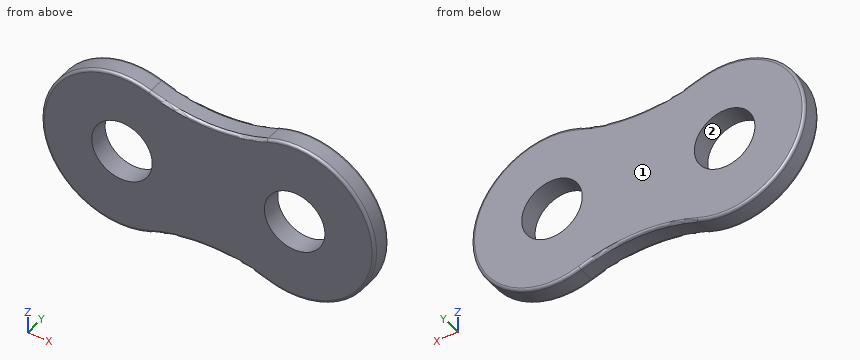
```python
from build123d import *

# Parameters (mm, degrees)
SZKIC1_R                    = 2.225
DODANIE_WYCI_GNI_CIE1_DEPTH = 1.5
ZAOKR_GLENIE1_R             = 0.2


with BuildPart() as part:
    # Szkic1 → Dodanie-wyciągnięcie1 (new body)
    with BuildSketch(Plane(origin=(0, 0, 0), x_dir=(1, 0, 0), z_dir=(0, 1, 0))):
        with BuildLine():
            ThreePointArc((2.036141304, 5.537520076), (-5.9, 0), (2.036141304, -5.537520076))
            ThreePointArc((2.036141304, -5.537520076), (6.35, -4.769554134), (10.663858696, -5.537520076))
            ThreePointArc((10.663858696, -5.537520076), (18.6, 0), (10.663858696, 5.537520076))
            ThreePointArc((10.663858696, 5.537520076), (6.35, 4.769554134), (2.036141304, 5.537520076))
        make_face()
        with Locations(Location((0, 0, 0), (0, 0, 270))):
            Circle(SZKIC1_R, mode=Mode.SUBTRACT)
        with Locations(Location((12.7, 0, 0), (0, 0, 270))):
            Circle(SZKIC1_R, mode=Mode.SUBTRACT)
    extrude(amount=DODANIE_WYCI_GNI_CIE1_DEPTH)

    # Zaokrąglenie1
    zaokr_glenie1_edges = [part.edges().sort_by_distance(p)[0] for p in [
        (6.35, 1.5, 4.769554134),
        (18.6, 1.5, 0),
        (6.35, 1.5, -4.769554134),
        (18.6, 0, 0),
        (6.35, 0, 4.769554134),
        (-5.9, 0, 0),
        (6.35, 0, -4.769554134),
        (-5.9, 1.5, 0),
    ]]
    fillet(zaokr_glenie1_edges, radius=ZAOKR_GLENIE1_R)


solid = part.part
```
Can you work these out from the model? Positions are in its coordinate system, mm. Face numbers are marked on the shaded views. Round coordinates to 2 decimals unless told otherwise and drop trailing zeros. Loops run counter-clockwise (first coordinate to the right, second up) from the corner with the lowest first, then second, coordinate; pieces in that order, holes last.
Item 1: Please list where these lines run through material, in increasing order: L1, parallel to X at y = 0.85, z = 0 (3 decimals); L2, parallel to Z at x = 13.5, y = 1.2; L3, parallel to Z at x = 13.75, y = 0.5.
Item 2: If we mould it in two halves opening along X, with no side actions, what happens to the marked faces 1 and 2? For each: +X half, -X half, draft (parallel to the pull), parting line (faces both ways), or undercut.
Item 3: Suppose I cut it at A-A, the plane y = 1. Write out the boundary of the cut face in (x, z) (3 decimals).
Item 4: Will these pins go through, and if not, where does the flat tip stop? pin 1 Ø6 at (x, z) = (4, -1.5) entering from -Y; pin 2 Ø2.5 at (x, z) = (0, 0) entering from +Y.
Item 5: Suppose I cut it at C-C, the plane z = -1.5. State how many separate pieces and enclosed holes the cut face has, then the cut area to 3 significant figures.
Item 6: Suppose I cut it at B-B, the plane z = 0. Write out the boundary of the cut face in (x, y) (3 decimals).
Reported:
1. L1: x = -5.9 to -2.225, 2.225 to 10.475, 14.925 to 18.6
1. L2: z = -5.85 to -2.08, 2.08 to 5.85
1. L3: z = -5.81 to -1.96, 1.96 to 5.81
2. face 1: draft
2. face 2: undercut
3. outline: (2.036, -5.538) arc R12.5 cw to (10.664, -5.538) arc R5.9 ccw (long way) to (10.664, 5.538) arc R12.5 cw to (2.036, 5.538) arc R5.9 ccw (long way) to start; hole circle Ø4.45 at (0, 0); hole circle Ø4.45 at (12.7, 0)
4. pin 1: stops at y = 0
4. pin 2: passes through
5. separate pieces: 3
5. enclosed holes: 0
5. area: 26.3 mm2
6. outline: (-5.9, 0.2) arc R0.2 ccw to (-5.7, 0) - (-2.225, 0) - (-2.225, 1.5) - (-5.7, 1.5) arc R0.2 ccw to (-5.9, 1.3) - close; (2.225, 0) - (10.475, 0) - (10.475, 1.5) - (2.225, 1.5) - close; (14.925, 0) - (18.4, 0) arc R0.2 ccw to (18.6, 0.2) - (18.6, 1.3) arc R0.2 ccw to (18.4, 1.5) - (14.925, 1.5) - close
